Geometry: final body of the model. Coordinates: model frame, mm. Face numbers are marked on the shaded views. Round coordinates to 2 decimals unless told otherwise and drop trailing zeros. Loops run counter-clockwise (first coordinate to the right, second up) from the corner with the lowest first, then second, coordinate; pieces in that order, holes last. Notation, with made-up numbers: M 65.5,74 L 94.5,74 A13 cw 94.5,80 Z; hole C 31,-25 d10. An arc over 180 degrees is marked long. Return JSON: item names as keys, results as strings.
Autodesk Inventor part; units mm, degrees
ref_plane "YZ Plane" through (0, 0, 0) normal (1, 0, 0) x (0, 1, 0)
ref_plane "XZ Plane" through (0, 0, 0) normal (0, 1, 0) x (-1, 0, 0)
ref_plane "XY Plane" through (0, 0, 0) normal (0, 0, 1) x (1, 0, 0)
sketch "Sketch1" plane through (0, 0, 0) normal (0, 0, 1) x (1, 0, 0)
  circle A0 centre (0, 0) radius 45
  circle A1 centre (0, 0) radius 35
  dimension "d0" = 70
  dimension "d2" = 90
extrude "Extrusion1" add sketch "Sketch1" along normal blind 8
sketch "Sketch2" plane through (0, 0, 8) normal (0, 0, 1) x (1, 0, 0)
  circle A0 centre (0, 0) radius 35
  circle A1 centre (0, 40) radius 1.75
  dimension "d5" = 40
  dimension "d6" = 3.5
extrude "Extrusion2" cut sketch "Sketch2" against normal through all contours A1
sketch "Sketch3" plane through (0, 0, 8) normal (0, 0, 1) x (1, 0, 0)
  circle A0 centre (0, 40) radius 1.75
  line L0 (3.1754, 40) -> (1.5877, 37.25)
  line L1 (1.5877, 37.25) -> (-1.5877, 37.25)
  line L2 (-1.5877, 37.25) -> (-3.1754, 40)
  line L3 (-3.1754, 40) -> (-1.5877, 42.75)
  line L4 (-1.5877, 42.75) -> (1.5877, 42.75)
  line L5 (1.5877, 42.75) -> (3.1754, 40)
  point P0 (0, 42.75)
  dimension "d9" = 5.5
extrude "Extrusion3" cut sketch "Sketch3" against normal blind 4
pattern_circular "Circular Pattern1" count 4 over 360 about axis through (0, 0, 0) along (0, 0, 1) of "Extrusion3", "Extrusion2"
properties part number "ring"
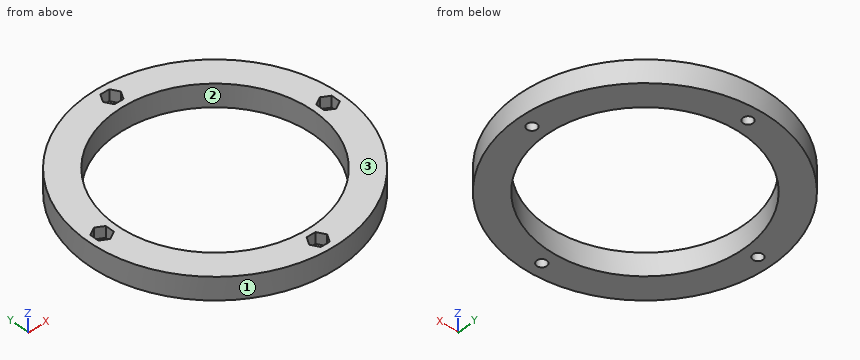
Q1. Section query C-C (y = -5.5). Output: boundary loops of the cut face in (x, z).
Determined:
{"outline": "M -44.66,0 L -34.57,0 L -34.57,8 L -44.66,8 Z; M 34.57,0 L 44.66,0 L 44.66,8 L 34.57,8 Z"}
Q2. Pull-direction query (Y, two-part tool) for the marked faces 1, 2 and 3; classes: pulls with the +Y half, pulls with the -Y half, needs draft (parallel to the pull), parting line crosses it, or undercut.
Determined:
{"face 1": "parting line crosses it", "face 2": "undercut", "face 3": "needs draft"}
Q3. Section query B-B (x = 0). Output: boundary loops of the cut face in (y, z), plus the area to 3 significant figures.
Determined:
{"outline": "M -45,0 L -41.75,0 L -41.75,4 L -42.75,4 L -42.75,8 L -45,8 Z; M -38.25,0 L -35,0 L -35,8 L -37.25,8 L -37.25,4 L -38.25,4 Z; M 35,0 L 38.25,0 L 38.25,4 L 37.25,4 L 37.25,8 L 35,8 Z; M 41.75,0 L 45,0 L 45,8 L 42.75,8 L 42.75,4 L 41.75,4 Z", "area": "88.0 mm^2"}
Q4. Section query A-A (z = 6). Output: boundary loops of the cut face in (x, y).
Determined:
{"outline": "C 0,0 d90; hole M -42.75,-1.59 L -40,-3.18 L -37.25,-1.59 L -37.25,1.59 L -40,3.18 L -42.75,1.59 Z; hole C 0,0 d70; hole M -3.18,-40 L -1.59,-42.75 L 1.59,-42.75 L 3.18,-40 L 1.59,-37.25 L -1.59,-37.25 Z; hole M -3.18,40 L -1.59,37.25 L 1.59,37.25 L 3.18,40 L 1.59,42.75 L -1.59,42.75 Z; hole M 37.25,-1.59 L 40,-3.18 L 42.75,-1.59 L 42.75,1.59 L 40,3.18 L 37.25,1.59 Z"}
Q5. Pin query (flat end, axial travel): pin 1 (1 mm diameter, centred on y = 0.5, z = 6, fed in from -X); pin 2 (3 mm diameter, centred on x = -1, y = -40, fed in from +Z); pin 3 (3.5 mm diameter, centred on x = -0.5, z = 5.5, fed in from +Y); pin 4 (4 mm diameter, centred on y = 31.5, z = 3, fed in from -X). Return the tip coordinate at first contact, or that it passes through.
Determined:
{"pin 1": "stops at x = -45", "pin 2": "stops at z = 4", "pin 3": "stops at y = 45", "pin 4": "stops at x = -33.98"}
Q6. Material intervals for L1, parallel to Y at x = 0, z = 5.75; L2, parallel to X at y = -1.5, z = 2.75 (3 decimals); L3, parallel to X at y = -32, z = 6, sorted ascending.
Determined:
{"L1": "y = -45 to -42.75, -37.25 to -35, 35 to 37.25, 42.75 to 45", "L2": "x = -44.975 to -40.901, -39.099 to -34.968, 34.968 to 39.099, 40.901 to 44.975", "L3": "x = -31.64 to -14.18, 14.18 to 31.64"}
Q7. Section query D-D (x = -17). Output: boundary loops of the cut face in (y, z).
Determined:
{"outline": "M -41.67,0 L -30.59,0 L -30.59,8 L -41.67,8 Z; M 30.59,0 L 41.67,0 L 41.67,8 L 30.59,8 Z"}
